CAD build for the part. Positions are in the model's coordinates, mm. Face numbers are marked on the shaded views. A direction names the side the tool comes from. Round coordinates to 2 decimals unless told otherwise and drop trailing zeros. Loops run counter-clockwise (first coordinate to the right, second up) from the corner with the lowest first, then second, coordinate; pieces in that order, holes last.
```python
from build123d import *

# Parameters (mm, degrees)
SKETCH1_R               = 4
BOSS_EXTRUDE1_DEPTH     = 6
SKETCH2_R               = 7
BOSS_EXTRUDE2_DEPTH     = 2
LPATTERN1_COUNT         = 2
LPATTERN1_PITCH         = 14
CUT_EXTRUDE1_DEPTH      = 13.727922061
CUT_EXTRUDE1_DEPTH_BACK = 13.727922061
SKETCH3_R               = 2.5
CHAMFER1_SIZE           = 1


with BuildPart() as part:
    # Sketch1 → Boss-Extrude1 (new, symmetric)
    with BuildSketch(Plane.XY):
        Circle(SKETCH1_R)
    extrude(amount=BOSS_EXTRUDE1_DEPTH, both=True)

    # Sketch2 → Boss-Extrude2 (add)
    with BuildSketch(Plane.XY.offset(6)):
        Circle(SKETCH2_R)
    boss_extrude2 = extrude(amount=BOSS_EXTRUDE2_DEPTH)

    # LPattern1: Boss-Extrude2 ×2
    with Locations(*[(0, 0, -i * LPATTERN1_PITCH) for i in range(1, LPATTERN1_COUNT)]):
        add(boss_extrude2)

    # Sketch3 → Cut-Extrude1 (cut, two sides: drawn at the far end of the back side and taken through both)
    with BuildSketch(Plane.XY.offset(-CUT_EXTRUDE1_DEPTH_BACK)):
        Circle(SKETCH3_R)
    extrude(amount=CUT_EXTRUDE1_DEPTH + CUT_EXTRUDE1_DEPTH_BACK, mode=Mode.SUBTRACT)

    # Chamfer1
    chamfer1_edges = [part.edges().sort_by_distance(p)[0] for p in [
        (-7, 0, 8),
        (-7, 0, -8),
    ]]
    chamfer(chamfer1_edges, length=CHAMFER1_SIZE)


solid = part.part
```
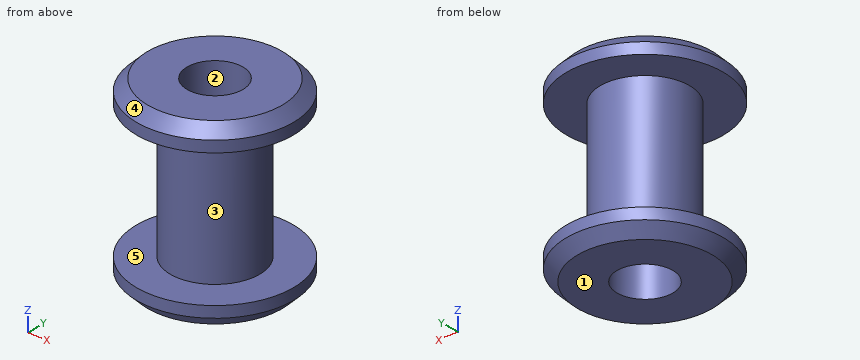
Item 1: Cut at C-C, the plane z = -3.25. Give the cut face in (x, y).
Answers follow:
outline: circle Ø8 at (0, 0); hole circle Ø5 at (0, 0)
Item 2: Probe line 1 (Z direction, x = -3, y = -3.5); line 2 (Y direction, x = 0, z = 1.5); line 3 (Y direction, x = -0.75, z = 5.5). List the from-to ranges inside material, lowest first.
Answers follow:
line 1: z = -8 to -6, 6 to 8
line 2: y = -4 to -2.5, 2.5 to 4
line 3: y = -3.93 to -2.38, 2.38 to 3.93
Item 3: Two-plate mould, pull along Z, no slides. Class the marked faces 1, 2 and 3: released by +Z, released by -Z, zero draft, split by the parting line, or undercut.
Answers follow:
face 1: released by -Z
face 2: zero draft
face 3: undercut
Item 4: Flat gauge pins, fed straight in: P1, Ø5, axis at y = -5.5, z = 2.5, coming from the -X side; P2, Ø8, axis at y = 1, z = -3.5, coming from the +X side; P3, Ø1, axis at y = -2, z = -1, coming from the -X side; P4, Ø5, axis at x = 3, z = 1.5, coming from the -Y side. Where does each tip first touch, or does it go through?
Answers follow:
P1: stops at x = -2.65
P2: stops at x = 7
P3: stops at x = -3.71
P4: stops at y = -3.97
Item 5: 3-axis set-ups, long thin cutter, end or side, ignore diameter. For the marked faces 4 and 5: which of +Z, -Z, +X, -X, +Y, -Y reach the whole face in a straight line?
Answers follow:
face 4: +Z
face 5: none
Item 6: Cut at A-A, the plane y = 0. Give the cut face in (x, z).
Answers follow:
outline: (-7, -7) - (-6, -8) - (-2.5, -8) - (-2.5, 8) - (-6, 8) - (-7, 7) - (-7, 6) - (-4, 6) - (-4, -6) - (-7, -6) - close; (2.5, -8) - (6, -8) - (7, -7) - (7, -6) - (4, -6) - (4, 6) - (7, 6) - (7, 7) - (6, 8) - (2.5, 8) - close
